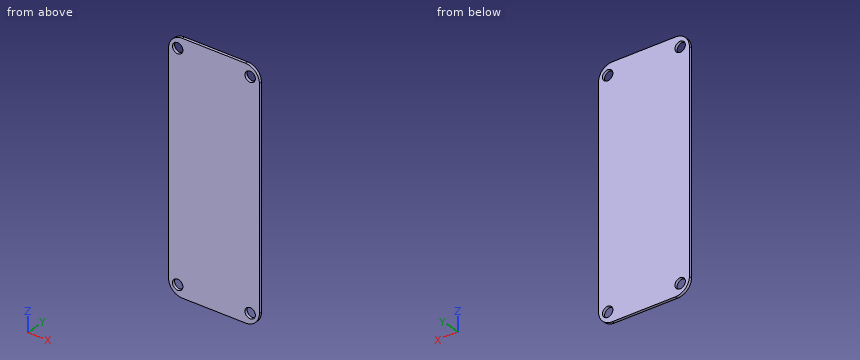
Autodesk Inventor part; units mm, degrees
ref_plane "YZ Plane" through (0, 0, 0) normal (1, 0, 0) x (0, 1, 0)
ref_plane "XZ Plane" through (0, 0, 0) normal (0, 1, 0) x (-1, 0, 0)
ref_plane "XY Plane" through (0, 0, 0) normal (0, 0, 1) x (1, 0, 0)
sketch "Sketch1" plane through (0, 0, 0) normal (0, 1, 0) x (-1, 0, 0)
  line L0 (0, 0) -> (39.5, 0)
  line L1 (39.5, 0) -> (39.5, -104.35)
  line L2 (39.5, -104.35) -> (0, -104.35)
  line L3 (0, -104.35) -> (0, 0)
  dimension "d0" = 104.35
  dimension "d1" = 39.5
extrude "Extrusion1" add sketch "Sketch1" along normal blind 1.2
fillet "Fillet1" radius 6 4 edges at (0, 0.6, 0) (-39.5, 0.6, 0) (0, 0.6, -104.35) (-39.5, 0.6, -104.35)
sketch "Sketch2" plane through (0, 0, 0) normal (0, -1, 0) x (1, 0, 0)
  line L0 (-35.5, -99.675) -> (-4, -99.675) construction
  line L1 (-4, -99.675) -> (-4, -4.675) construction
  line L2 (-4, -4.675) -> (-35.5, -4.675) construction
  line L3 (-35.5, -4.675) -> (-35.5, -99.675) construction
  line L4 (0, -98.35) -> (0, -6) construction
  line L5 (-39.5, -6) -> (-39.5, -98.35) construction
  line L6 (-6, 0) -> (-33.5, 0) construction
  line L7 (-33.5, -104.35) -> (-6, -104.35) construction
  point P0 (0, 0)
  dimension "d5" = 95
  dimension "d6" = 31.5
  dimension "d7" = 39.5
  dimension "d8" = 4
  dimension "d9" = 104.35
  dimension "d10" = 4.675
hole "Hole1" at (-35.5, 0, -99.675) at (-4, 0, -99.675) at (-4, 0, -4.675) at (-35.5, 0, -4.675) direction (0, 1, 0) diameter 4.5 depth 1.2
equation "\"d8\" = -0.5 * d6 + 0.5 * d7"
equation "\"d10\" = -0.5 * d5 + 0.5 * d9"
properties part number "PCB"
Source: CAD feature listing. Evaluate the final solid. Frame: model axes, mm. Round coordinates to 2 decimals unless told otherwise and drop trailing zeros. Write each loop counter-clockwise with the first axis right and the second up, starting at its lowest first coordinate (ties: lowest second). Pieces come first, ordered by that corner, then holes. Notation, with made-up numbers: M -0.5,59.25 L 52.5,59.25 A8 ccw 52.5,69.25 Z; hole C -10.75,-13 d10. An arc over 180 degrees is marked long. Answer as a JSON object with one key per item and string values. Group by question number.
(1) Ray query, line 1 (Z direction, x = -35.5, y = 0.5) (3 decimals); line 2 (Z direction, x = -33.5, y = 0.2); line 3 (X direction, y = 1.1, z = -4). Return the intervals inside material, ascending. Write a range as [from, to].
(2) Section query B-B on x = -35.5. Output: boundary loops of the cut face in (y, z) (3 decimals).
(3) Section query A-A on y = 0.6. Output: boundary loops of the cut face in (x, z) (3 decimals).
(4) First-contact query: pin 1 (4 mm diameter, centred on x = -35.5, z = -4.675, fed in from -Y). Flat tip, straight axial feed; report the tip coordinate or a pass-through.
Computed values:
{
 "1": {"line 1": "[-104.007, -101.925], [-97.425, -6.925], [-2.425, -0.343]", "line 2": "[-104.35, -100.71], [-98.64, -5.71], [-3.64, 0]", "line 3": "[-39.16, -37.65], [-33.35, -6.15], [-1.85, -0.34]"},
 "2": {"outline": "M 0,-104.007 L 1.2,-104.007 L 1.2,-101.925 L 0,-101.925 Z; M 0,-97.425 L 1.2,-97.425 L 1.2,-6.925 L 0,-6.925 Z; M 0,-2.425 L 1.2,-2.425 L 1.2,-0.343 L 0,-0.343 Z"},
 "3": {"outline": "M -39.5,-98.35 A6 ccw -33.5,-104.35 L -6,-104.35 A6 ccw 0,-98.35 L 0,-6 A6 ccw -6,0 L -33.5,0 A6 ccw -39.5,-6 Z; hole C -35.5,-99.675 d4.5; hole C -35.5,-4.675 d4.5; hole C -4,-99.675 d4.5; hole C -4,-4.675 d4.5"},
 "4": {"pin 1": "through"}
}
